```python
from build123d import *

# Parameters (mm, degrees)
CROQUIS1_W              = 24
CROQUIS1_H              = 27
SALIENTE_EXTRUIR1_DEPTH = 25
SALIENTE_EXTRUIR2_DEPTH = 15
CROQUIS5_R              = 2
CORTAR_EXTRUIR1_DEPTH   = 27


with BuildPart() as part:
    # Croquis1 → Saliente-Extruir1 (new body)
    with BuildSketch(Plane.XY):
        with Locations((-37, 0.422764228)):
            Rectangle(CROQUIS1_W, CROQUIS1_H)
    extrude(amount=SALIENTE_EXTRUIR1_DEPTH)

    # Croquis2 → Saliente-Extruir2 (add)
    with BuildSketch(Plane(origin=(0, 13.922764228, 0), x_dir=(1, 0, 0), z_dir=(0, 1, 0))):
        with BuildLine():
            Line((-40.95, -8.35), (-33.05, -8.35))
            ThreePointArc((-33.05, -8.35), (-32.908578644, -8.408578644), (-32.85, -8.55))
            Line((-32.85, -8.55), (-32.85, -16.45))
            ThreePointArc((-32.85, -16.45), (-32.908578644, -16.591421356), (-33.05, -16.65))
            Line((-33.05, -16.65), (-40.95, -16.65))
            ThreePointArc((-40.95, -16.65), (-41.091421356, -16.591421356), (-41.15, -16.45))
            Line((-41.15, -16.45), (-41.15, -8.55))
            ThreePointArc((-41.15, -8.55), (-41.091421356, -8.408578644), (-40.95, -8.35))
        make_face()
    extrude(amount=SALIENTE_EXTRUIR2_DEPTH)

    # Croquis5 → Cortar-Extruir1 (cut)
    with BuildSketch(Plane(origin=(0, 13.922764228, 0), x_dir=(1, 0, 0), z_dir=(0, 1, 0))):
        with Locations(Location((-46.551489219, -22.396688282, 0), (0, 0, 270))):
            Circle(CROQUIS5_R)
        with Locations(Location((-28, -21.888198758, 0), (0, 0, 270))):
            Circle(CROQUIS5_R)
        with Locations(Location((-46, -3.267515924, 0), (0, 0, 270))):
            Circle(CROQUIS5_R)
        with Locations(Location((-28, -3.111801242, 0), (0, 0, 270))):
            Circle(CROQUIS5_R)
    extrude(amount=-CORTAR_EXTRUIR1_DEPTH, mode=Mode.SUBTRACT)


solid = part.part
```
Check sheet for the modelled part. Datum: model origin and axes. Units: mm. A direction names the side the tool comes from. Give positions to 0.01 mm unless a question says otherwise; leave off trailing zeros. Order: outer loops, then holes, each group sorted by start corner. A loop starts at its lowest first (then second) coordinate and runs counter-clockwise, first axis right, second up. Notation, with made-up numbers: M -8,-31.75 L 50,-31.75 A22 cw 50,7.25 Z; hole C 36,56 d1. An arc over 180 degrees is marked long. Answer in a Markdown table with one row per item. Add a question column.
Q1. Thickness scan on L1, parallel to Z at x = -45, y = 12.5; L2, parallel to Z at x = -45.5, y = -6; L3, parallel to X at y = -0.5, z = 22.75. Record the ranges inside material, lowest first.
Q2. Sectioned sample at A-A, the plane x = -40. Record the boundary of the cut face in (y, z).
Q3. Release check for a two-part mould opening along Z. For faces 1 (the cylindrical face through (-29.952, 0.612, 2.678)), 2 (the flat face through (-43, 13.923, 12)), 3 (the flat face through (-37, 21, 16.65)), 4 (the flat face through (-37, 21, 8.35)) record: released by +Z, released by -Z, zero draft, split by the parting line, or undercut.
Q4. Access from +Z, -Z, +X, -X, +Y, -Y to the whole of each face (thin tool, end or side, straight path). Record for faces 5 (the flat face through (-41.15, 21, 13)), 6 (the flat face through (-32.85, 21, 12)), 7 (the flat face through (-49, 0, 12)).
Q5. Sectioned sample at C-C, the plane z = 11. Record the boundary of the cut face in (x, y).
Q6. Gauge pin test, flat ends, axial feed: pin 1 Ø8.5 at (y, z) = (20.5, 13.5) entering from +X; pin 2 Ø5 at (x, z) = (-28, 21.89) entering from +Y; pin 3 Ø3.5 at (x, z) = (-28, 3.11) entering from +Y; pin 4 Ø6.5 at (x, y) = (-36.5, 23.5) entering from -Z. Record the tip position at first contact, or that the pin passes through.
Q7. Sectioned sample at B-B, the plane x = -28. Record the boundary of the cut face in (y, z), and give its area (3 significant figures).
Q8. Sectioned sample at D-D, the plane y = 8. Record the boundary of the cut face in (x, z).
Verdict:
| question | item | result |
|---|---|---|
| 1 | L1 | 0 to 1.54, 5 to 21.13, 23.66 to 25 |
| 1 | L2 | 0 to 1.33, 5.2 to 20.7, 24.1 to 25 |
| 1 | L3 | -49 to -48.52, -44.58 to -29.8, -26.2 to -25 |
| 2 | outline | M -13.08,0 L 13.92,0 L 13.92,8.35 L 28.92,8.35 L 28.92,16.65 L 13.92,16.65 L 13.92,25 L -13.08,25 Z |
| 3 | face 1 | undercut |
| 3 | face 2 | zero draft |
| 3 | face 3 | released by +Z |
| 3 | face 4 | released by -Z |
| 4 | face 5 | +Z, -Z, -X, +Y |
| 4 | face 6 | +Z, -Z, +X, +Y |
| 4 | face 7 | +Z, -Z, -X, +Y, -Y |
| 5 | outline | M -49,-13.08 L -25,-13.08 L -25,13.92 L -32.85,13.92 L -32.85,28.92 L -41.15,28.92 L -41.15,13.92 L -49,13.92 Z |
| 6 | pin 1 | x = -32.85 |
| 6 | pin 2 | y = 13.92 |
| 6 | pin 3 | through |
| 6 | pin 4 | z = 8.35 |
| 7 | outline | M -13.08,0 L 13.92,0 L 13.92,1.11 L -13.08,1.11 Z; M -13.08,5.11 L 13.92,5.11 L 13.92,19.89 L -13.08,19.89 Z; M -13.08,23.89 L 13.92,23.89 L 13.92,25 L -13.08,25 Z |
| 7 | area | 459 mm² |
| 8 | outline | M -49,0 L -25,0 L -25,25 L -49,25 Z; hole C -46.55,22.4 d4; hole C -46,3.27 d4; hole C -28,3.11 d4; hole C -28,21.89 d4 |
